from build123d import *


with BuildPart() as part:
    # Sketch1 → Revolve1 (revolve)
    with BuildSketch(Plane.XY):
        Polygon((-44.45, 0), (-44.45, 76.2), (-38.1, 76.2), (-12.7, 61.535303163), (-12.7, 55.185303163), (-28.321, 0), align=None)
    revolve(axis=Axis((0, 0, 0), (0, 1, 0)))

    # Sketch2 → Cut-Revolve1 (revolve, cut)
    with BuildSketch(Plane.XY):
        with BuildLine():
            Line((-44.45, 57.15), (-39.624, 57.15))
            ThreePointArc((-39.624, 57.15), (-39.444394878, 57.075605122), (-39.37, 56.896))
            Line((-39.37, 56.896), (-39.37, 51.816))
            ThreePointArc((-39.37, 51.816), (-39.444394878, 51.636394878), (-39.624, 51.562))
            Line((-39.624, 51.562), (-44.45, 51.562))
            Line((-44.45, 51.562), (-44.45, 57.15))
        make_face()
    revolve(axis=Axis((0, 0, 0), (0, 1, 0)), mode=Mode.SUBTRACT)


solid = part.part
Part model, mm, in its own coordinate system. A direction names the side the tool comes from. Round coordinates to 2 decimals unless told otherwise and drop trailing zeros. Order: outer loops, then holes, each group sorted by start corner. A loop starts at its lowest first (then second) coordinate and runs counter-clockwise, first axis right, second up. Notation, with made-up numbers: (-9.5, -22.5) -> (29.5, -22.5) arc R18 ccw to (29.5, -5.5) -> close; hole circle Ø5 at (-39, 43). An arc over 180 degrees is marked (long way). Put each result on its own line as item: value.
Q1. Wall check: line 1 (Z direction, x = 0, y = 59); line 2 (Y direction, x = -24.5, z = -31); line 3 (Y direction, x = 28, z = 32). Give the ranges that are in metal, low to high. Write a range as [from, to].
From the geometry:
line 1: z = [-44.45, -12.7], [12.7, 44.45]
line 2: y = [0, 51.59], [57.12, 76.2]
line 3: y = [0, 51.56], [57.15, 76.2]
Q2. Band-saw the part on D-D (y = 60). Give the cut face in (x, z), and give its area (3 significant figures).
From the geometry:
outline: circle Ø88.9 at (0, 0); hole circle Ø25.4 at (0, 0)
area: 5,700 mm2
Q3. Band-saw the part on A-A (z = 0). Give the cut face in (x, y), and give its area (3 significant figures).
From the geometry:
outline: (-44.45, 0) -> (-28.32, 0) -> (-12.7, 55.19) -> (-12.7, 61.54) -> (-38.1, 76.2) -> (-44.45, 76.2) -> (-44.45, 57.15) -> (-39.62, 57.15) arc R0.25 cw to (-39.37, 56.9) -> (-39.37, 51.82) arc R0.25 cw to (-39.62, 51.56) -> (-44.45, 51.56) -> close; (12.7, 55.19) -> (28.32, 0) -> (44.45, 0) -> (44.45, 51.56) -> (39.62, 51.56) arc R0.25 cw to (39.37, 51.82) -> (39.37, 56.9) arc R0.25 cw to (39.62, 57.15) -> (44.45, 57.15) -> (44.45, 76.2) -> (38.1, 76.2) -> (12.7, 61.54) -> close
area: 3,550 mm2
Q4. Pin check, flat tips, straight feed: pin 1 Ø1.5 at (y, z) = (17.5, 13) entering from -X; pin 2 Ø4 at (x, y) = (8.5, 15.5) entering from +Z; pin 3 Ø1.5 at (x, y) = (-30.5, 18) entering from +Z; pin 4 Ø15 at (x, z) = (0, 0) entering from +Y. Stop position of each tip, or through.
From the geometry:
pin 1: stops at x = -42.73
pin 2: stops at z = 43.97
pin 3: stops at z = 33.03
pin 4: passes through
Q5. Band-saw the part on C-C (y = 34.5). Give the cut face in (x, z), and give its area (3 significant figures).
From the geometry:
outline: circle Ø88.9 at (0, 0); hole circle Ø37.11 at (0, 0)
area: 5,130 mm2
Q6. Pull direction Y, two halves, no side cores. Call faces 3 (the face through (2.75, 58.32, -12.4)), 4 (the face through (31.24, 54.32, -23.96)), 5 (the face through (3.02, 62.247, -13.602)): pulls with the +Y half, pulls with the -Y half, needs draft (parallel to the pull), parting line crosses it, or undercut.
From the geometry:
face 3: needs draft
face 4: undercut
face 5: pulls with the +Y half
Q7. Band-saw the part on B-B (x = 0). Give the cut face in (y, z).
From the geometry:
outline: (0, -44.45) -> (51.56, -44.45) -> (51.56, -39.62) arc R0.25 cw to (51.82, -39.37) -> (56.9, -39.37) arc R0.25 cw to (57.15, -39.62) -> (57.15, -44.45) -> (76.2, -44.45) -> (76.2, -38.1) -> (61.54, -12.7) -> (55.19, -12.7) -> (0, -28.32) -> close; (0, 28.32) -> (55.19, 12.7) -> (61.54, 12.7) -> (76.2, 38.1) -> (76.2, 44.45) -> (57.15, 44.45) -> (57.15, 39.62) arc R0.25 cw to (56.9, 39.37) -> (51.82, 39.37) arc R0.25 cw to (51.56, 39.62) -> (51.56, 44.45) -> (0, 44.45) -> close
Q8. Tool access for faces 1 (the face through (-40, 51.562, -3)), 2 (the face through (-42.397, 26.142, 13.352)): list every direction of +Z, -Z, +X, -X, +Y, -Y with a clear straight run to the whole face (end or side of a thin tool).
From the geometry:
face 1: none
face 2: +Y, -Y
